For this review, take the finished solid that the model builds, in its own axes (mm). Face numbers are marked on the shaded views. A direction names the side the tool comes from. Round coordinates to 2 decimals unless told otherwise and drop trailing zeros. Order: outer loops, then holes, each group sorted by start corner. A loop starts at its lowest first (then second) coordinate and runs counter-clockwise, first axis right, second up. Notation, with made-up numbers: (-18.75, 5) - (1.25, 5) arc R30 ccw to (1.25, 29) - close; hole circle Ø9 at (-1, 61.5). An arc over 180 degrees is marked (long way). One line per question, with ' | ' between items.
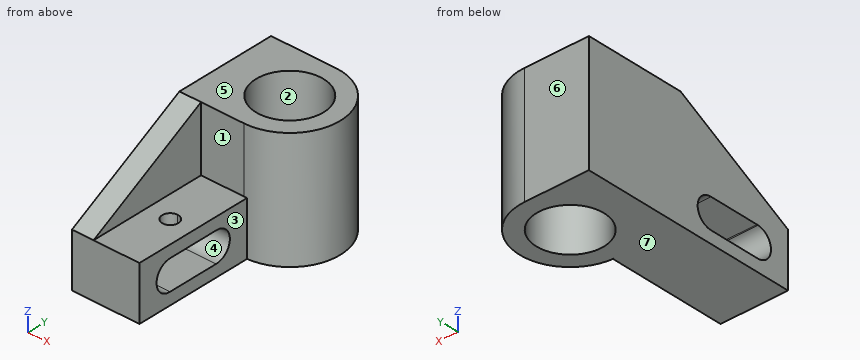
```python
from build123d import *

# Parameters (mm, degrees)
F0_R     = 25
F1_DEPTH = 88
F2_W     = 88
F2_H     = 40
F3_DEPTH = 50
F5_DEPTH = 16
F7_DEPTH = 9.008194986


with BuildPart() as f1:
    # F0 (on Top) → F1 (new body)
    with BuildSketch(Plane.XY):
        with BuildLine():
            Line((0, 75), (0, 0))
            Line((0, 0), (47.7671325207, 0))
            ThreePointArc((47.7671325207, 0), (85.2671325207, 37.5), (47.7671325207, 75))
            Line((47.7671325207, 75), (0, 75))
        make_face()
        with Locations((47.7671325207, 37.5)):
            Circle(F0_R, mode=Mode.SUBTRACT)
    extrude(amount=F1_DEPTH)

    # F2 (on Right) → F3 (join)
    with BuildSketch(Plane.YZ):
        with Locations((-44, 20)):
            Rectangle(F2_W, F2_H)
        with BuildLine():
            ThreePointArc((-63.4935666774, 30.9889213272), (-63.0031659942, 30.9999995444), (-62.5127590152, 30.989203621))
            Line((-62.5127590152, 30.989203621), (-25.0031659942, 30.9999995444))
            ThreePointArc((-25.0031659942, 30.9999995444), (-14.0013797727, 19.8257786016), (-25.3515634815, 9.0056194755))
            Line((-25.3515634815, 9.0056194755), (-62.9983580838, 9.0000001225))
            ThreePointArc((-62.9983580838, 9.0000001225), (-62.9991790419, 9.0000000306), (-63, 9))
            ThreePointArc((-63, 9), (-73.997229983, 19.7531545007), (-63.4935666774, 30.9889213272))
        make_face(mode=Mode.SUBTRACT)
    extrude(amount=F3_DEPTH)

    # F4 (on Right) → F5 (join)
    with BuildSketch(Plane.YZ):
        Polygon((-88, 40), (0, 40), (0, 88), align=None)
    extrude(amount=F5_DEPTH)

    # F6 (on face) → F7 (cut, through all)
    with BuildSketch(Plane.XY.offset(40)):
        with BuildLine():
            ThreePointArc((39, -44), (37.2426406871, -39.7573593129), (33, -38))
            ThreePointArc((33, -38), (28.7573593129, -48.2426406871), (39, -44))
        make_face()
    extrude(amount=-F7_DEPTH, mode=Mode.SUBTRACT)


solid = f1.part
```
(1) We need section D-D on y = -46.5. State the section outline as (x, z) points.
Output values:
outline: (0, 0) - (50, 0) - (50, 9) - (0, 9) - close; (0, 30.99) - (27.55, 30.99) - (27.55, 40) - (16, 40) - (16, 62.64) - (0, 62.64) - close; (38.45, 30.99) - (50, 30.99) - (50, 40) - (38.45, 40) - close
(2) Insertion check: pin 1 (12 mm diameter, centred on x = 55.5, y = -52, fed in from -Z); pin 2 (20 mm diameter, centred on y = -31, z = 12.5, fed in from +X); pin 3 (14.5 mm diameter, centred on y = -50, z = 67.5, fed in from +X); pin 4 (10 mm diameter, centred on x = 39.5, y = -66, fed in from +Z). Each pin has a flat end and moves straight along its axis. Give the tip position at first contact, or say it passes through.
Output values:
pin 1: z = 0 | pin 2: x = 50 | pin 3: x = 16 | pin 4: z = 40
(3) Mouldability with a two-part tool opening along Z and no side actions: class the marked faces 4, 5, 6 and 7 as released by +Z, released by -Z, zero draft, split by the parting line, or undercut.
Output values:
face 4: undercut | face 5: released by +Z | face 6: zero draft | face 7: released by -Z
(4) For probe 1 along Z at (x, y) = (42.5, -64); probe 2 along X at (y, z) = (-44, 35); probe 3 along Y at (x, z) = (33, 37.5), list the stretches that pass through material, from the lowest coordinate up. Write a range as [from, to].
Output values:
probe 1: [0, 9.05], [30.95, 40] | probe 2: [0, 27], [39, 50] | probe 3: [-88, -50], [-38, 17.33], [57.67, 75]
(5) For the marked faces 1, 2 and 3, list the 3-axis set-ups (+Z, -Z, +X, -X, +Y, -Y) from which the entire face can be reached by the end or side of a thin tool; tool diameter is ignored.
Output values:
face 1: +Z, +X, -Y | face 2: +Z, -Z | face 3: +Z, -Z, +X, -Y
(6) We need section C-C on z = 55. State the section outline as (x, y) points, plus the area to 3 significant figures.
Output values:
outline: (0, -60.5) - (16, -60.5) - (16, 0) - (47.77, 0) arc R37.5 ccw to (47.77, 75) - (0, 75) - close; hole circle Ø50 at (47.77, 37.5) | area: 4,800 mm^2
(7) We need section A-A on y = 37.5. State the section outline as (x, z) points.
Output values:
outline: (0, 0) - (22.77, 0) - (22.77, 88) - (0, 88) - close; (72.77, 0) - (85.27, 0) - (85.27, 88) - (72.77, 88) - close
